Source: three-view drawing plus pictorial views. Frame: mm from the lowest corner of the part. A direction names the side the tool comes from. Give positions to 0.01 mm unless a question says otherwise; leave off trailing zeros. Loops run counter-clockwise (first coordinate to the right, second up) from the corner with the lowest first, then second, coordinate; pieces in that order, holes last.
1. Section D-D, the plane y = 12.5. Output: boundary loops of the cut face in (x, z), then the cut area to 3 significant figures.
2. Section A-A, the plane z = 1.5. Output: boundary loops of the cut face in (x, y), then the cut area to 3 significant figures.
3. First-contact query: P1, Ø1, axis at y = 33.5, z = 1, coming from the -X side; P2, Ø3, axis at x = 11, y = 31.5, coming from the -Z side; P3, Ø2, axis at y = 26, z = 1, coming from the -X side (1 decimal). Flat tips, straight axial feed; report the tip coordinate or a pass-through.
4. Section B-B, the plane z = 3.75. Output: boundary loops of the cut face in (x, y).
5. Section C-C, the plane x = 16.25. Output: boundary loops of the cut face in (y, z).
6. Access query for the marked faces 1 and 2. Directions: +Z, -Z, +X, -X, +Y, -Y. A direction counts if a zero-diameter tool reaches every point of the face in a straight line with its end or side. Return the directions, or none.
7. Material intervals for line 1 along X through (y, z) = (6.5, 0.5); line 2 along Y through (x, z) = (20.5, 1); line 3 along Y through (x, z) = (2.5, 2.75) (1 decimal), sorted ascending.
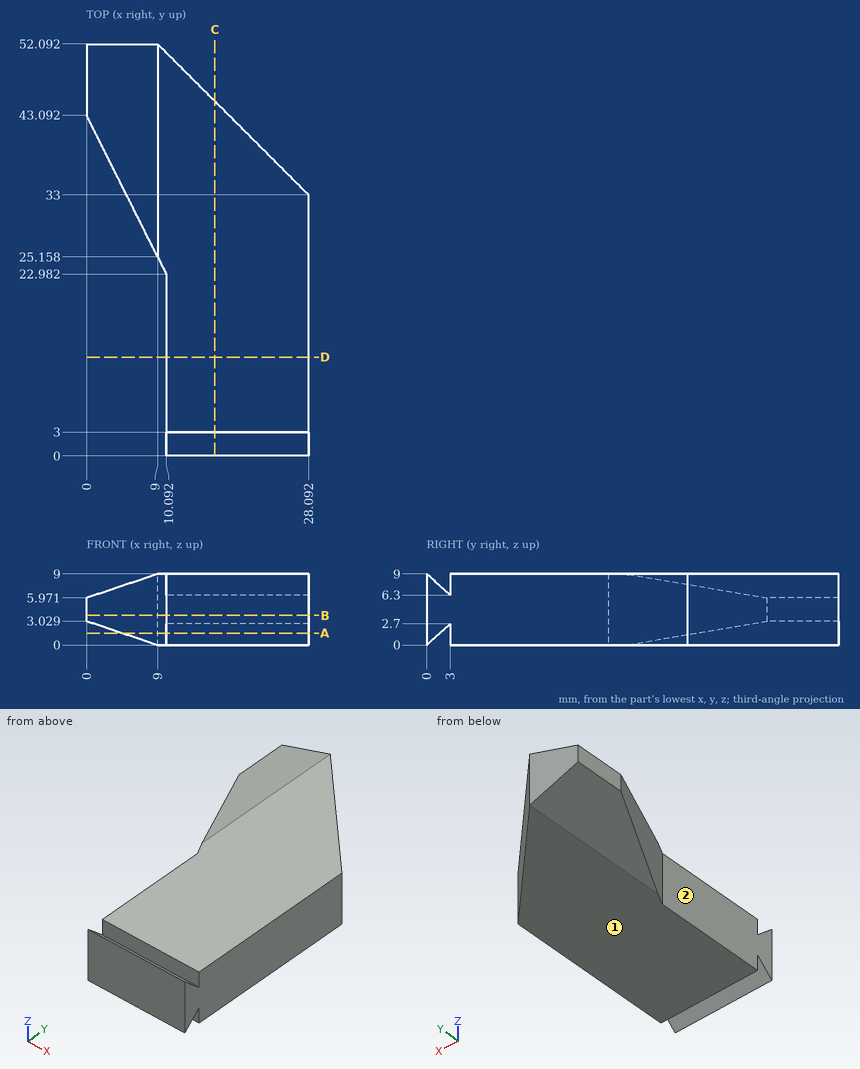
Answers below:
1. outline: (10.09, 0) - (28.09, 0) - (28.09, 9) - (10.09, 9) - close
1. area: 162 mm2
2. outline: (4.54, 34.04) - (10.09, 22.98) - (10.09, 3) - (28.09, 3) - (28.09, 33) - (9, 52.09) - (4.54, 52.09) - close; (10.09, 0) - (28.09, 0) - (28.09, 1.67) - (10.09, 1.67) - close
2. area: 862 mm2
3. P1: stops at x = 4.7
3. P2: stops at z = 0
3. P3: stops at x = 8.1
4. outline: (0, 43.09) - (10.09, 22.98) - (10.09, 0) - (28.09, 0) - (28.09, 33) - (9, 52.09) - (0, 52.09) - close
5. outline: (0, 0) - (3, 2.7) - (3, 0) - (44.84, 0) - (44.84, 9) - (3, 9) - (3, 6.3) - (0, 9) - close
6. face 1: -Z, +X, -X, +Y, -Y
6. face 2: +Z, -Z, -X, -Y
7. line 1: x = 10.09 to 28.09
7. line 2: y = 0 to 1.11, 3 to 40.59
7. line 3: y = 38.1 to 52.1
